from build123d import *

# Parameters (mm, degrees)
F0_R     = 14.2875
F1_DEPTH = 50.8
F3_R     = 7.874
F2_R     = 7.874
F4_DEPTH = 25.4
F6_DEPTH = 127
F8_DEPTH = 25.4


with BuildPart() as f1:
    # F0 (on Front) → F1 (new body)
    with BuildSketch(Plane.XZ):
        Polygon((0, 12.7), (0, 0), (133.096, 0), (133.096, 12.7), (94.985996, 12.7), (94.985996, 15.748), (38.274846, 15.748), (38.274846, 12.7), align=None)
        with BuildLine():
            Line((38.274846, 37.998795), (38.274846, 15.748))
            Line((38.274846, 15.748), (94.985996, 15.748))
            Line((94.985996, 15.748), (94.985996, 40.393602))
            Line((94.985996, 40.393602), (94.985996, 41.902398))
            ThreePointArc((94.985996, 41.902398), (67.748237, 69.570669), (38.274846, 44.297205))
            Line((38.274846, 44.297205), (38.274846, 37.998795))
        make_face()
        with Locations((66.548, 41.148)):
            Circle(F0_R, mode=Mode.SUBTRACT)
        with BuildLine():
            ThreePointArc((38.274846, 44.297205), (38.1, 41.148), (38.274846, 37.998795))
            Line((38.274846, 37.998795), (38.274846, 44.297205))
        make_face()
        with BuildLine():
            Line((94.985996, 41.902398), (94.985996, 40.393602))
            ThreePointArc((94.985996, 40.393602), (94.996, 41.148), (94.985996, 41.902398))
        make_face()
    extrude(amount=F1_DEPTH)

    # F3 (on face) + F2 (on face) → F4 (cut)
    with BuildSketch(Plane.XY.offset(12.7)):
        with Locations((114.040998, -25.4)):
            Circle(F3_R)
    with BuildSketch(Plane.XY.offset(12.7)):
        with Locations((19.137423, -25.4)):
            Circle(F2_R)
    extrude(amount=-F4_DEPTH, mode=Mode.SUBTRACT)

    # F5 (on face) → F6 (cut)
    with BuildSketch(Plane.YZ.offset(94.985996)):
        Polygon((-50.8, 68.641677), (-50.8, 15.748), (-29.999232, 72.897641), (-51.085521, 72.897641), align=None)
    extrude(amount=-F6_DEPTH, mode=Mode.SUBTRACT)

    # F7 (on face) → F8 (cut)
    with BuildSketch(Plane(origin=(94.985996, 0, 0), x_dir=(0, -1, 0), z_dir=(-1, 0, 0))):
        Polygon((50.8, 40.393602), (50.8, 41.902398), (41.280578, 41.902398), (41.829734, 40.393602), align=None)
    extrude(amount=-F8_DEPTH, mode=Mode.SUBTRACT)


solid = f1.part
Part model, mm, in its own coordinate system. A direction names the side the tool comes from. Round coordinates to 2 decimals unless told otherwise and drop trailing zeros. Loops run counter-clockwise (first coordinate to the right, second up) from the corner with the lowest first, then second, coordinate; pieces in that order, holes last. Notation, with made-up numbers: (16, 66) - (52, 66) arc R37 ccw to (52, 102) - close; hole circle Ø2 at (-19, 21). An arc over 180 degrees is marked (long way). Answer as a JSON object with one key per item and string values.
Item 1: Pin check, flat tips, straight feed: pin 1 (11.5 mm diameter, centred on x = 24.5, y = -17, fed in from +Z); pin 2 (6 mm diameter, centred on y = -40.5, z = 22.5, fed in from +X); pin 3 (3 mm diameter, centred on y = -40.5, z = 26, fed in from -X); pin 4 (12.5 mm diameter, centred on x = 114.04, y = -25.4, fed in from -Z). Stop position of each tip, or through.
Output:
{"pin 1": "z = 12.7", "pin 2": "x = 94.99", "pin 3": "x = 38.27", "pin 4": "through"}
Item 2: Band-saw the part on A-A on y = -21.5. List the corners of the cut face in (x, z) (1 decimal), plus the area to 3 significant figures.
Output:
{"outline": "(0, 0) - (12.3, 0) - (12.3, 12.7) - (0, 12.7) - close; (26, 0) - (107.2, 0) - (107.2, 12.7) - (95, 12.7) - (95, 40.4) arc R28.4 ccw to (95, 41.9) arc R28.4 ccw to (38.3, 44.3) arc R28.4 ccw to (38.3, 38) - (38.3, 12.7) - (26, 12.7) - close; (120.9, 0) - (133.1, 0) - (133.1, 12.7) - (120.9, 12.7) - close; hole circle Ø28.6 at (66.5, 41.1)", "area": "3,590 mm2"}
Item 3: Tool access for faces 1 (the face through (123, -25, 12.7)), 2 (the face through (133.096, -25, 6)): list every direction of +Z, -Z, +X, -X, +Y, -Y with a clear straight run to the whole face (end or side of a thin tool).
Output:
{"face 1": "+Z, +X, +Y, -Y", "face 2": "+Z, -Z, +X, +Y, -Y"}
Item 4: Band-saw the part on B-B on x = 25. List the corners of the cut face in (y, z).
Output:
{"outline": "(-50.8, 0) - (-30.66, 0) - (-30.66, 12.7) - (-50.8, 12.7) - close; (-20.14, 0) - (0, 0) - (0, 12.7) - (-20.14, 12.7) - close"}
Item 5: Wall check: L1, parallel to X at y = -27, z = 10.5; L2, parallel to X at y = -24, z = 4; L3, parallel to Z at x = 26.5, y = -46. Give the ranges that are in metal, low to high.
Output:
{"L1": "0 to 11.43, 26.85 to 106.33, 121.75 to 133.1", "L2": "0 to 11.39, 26.89 to 106.29, 121.79 to 133.1", "L3": "0 to 12.7"}
Item 6: Band-saw the part on C-C on z = 46.5. List the corners of the cut face in (x, y).
Output:
{"outline": "(38.61, -39.61) - (53.3, -39.61) - (53.3, 0) - (38.61, 0) - close; (79.8, -39.61) - (94.49, -39.61) - (94.49, 0) - (79.8, 0) - close"}
Item 7: Band-saw the part on D-D on y = -3.5. List the corners of the cut face in (x, z) (1 decimal), plus the area to 3 significant figures.
Output:
{"outline": "(0, 0) - (133.1, 0) - (133.1, 12.7) - (95, 12.7) - (95, 40.4) arc R28.4 ccw to (95, 41.9) arc R28.4 ccw to (38.3, 44.3) arc R28.4 ccw to (38.3, 38) - (38.3, 12.7) - (0, 12.7) - close; hole circle Ø28.6 at (66.5, 41.1)", "area": "3,930 mm2"}
Item 8: Pull direction Z, two halves, no side cores. Call faces 3 (the face through (66, -25, 0)), 4 (the face through (38.275, -25, 26)), 5 (the face through (121.55, -23.03, 6.44)): pulls with the +Z half, pulls with the -Z half, needs draft (parallel to the pull), parting line crosses it, or undercut.
Output:
{"face 3": "pulls with the -Z half", "face 4": "undercut", "face 5": "needs draft"}
